from build123d import *

# Parameters (mm, degrees)
F0_W     = 1.5875
F0_H     = 19.05
F1_DEPTH = 30.48
F2_DEPTH = 19.6596
F4_DEPTH = 10.8204


with BuildPart() as f1:
    # F0 (on Front) → F1 (new body)
    with BuildSketch(Plane.XZ):
        with Locations((-5.55625, 10.795)):
            Rectangle(F0_W, F0_H)
        Polygon((-4.7625, 1.27), (-6.35, 1.27), (-6.35, -1.27), (6.35, -1.27), (6.35, 1.27), (4.7625, 1.27), align=None)
        with Locations((5.55625, 10.795)):
            Rectangle(F0_W, F0_H)
    extrude(amount=F1_DEPTH)

    # F1_face (on face) → F2 (cut)
    with BuildSketch(Plane(origin=(0, -30.48, 7.040217), x_dir=(1, 0, 0), z_dir=(0, -1, 0))):
        Polygon((-6.35, 13.279783), (-6.35, -8.310217), (6.35, -8.310217), (6.35, 13.279783), (4.7625, 13.279783), (4.7625, -5.770217), (-4.7625, -5.770217), (-4.7625, 13.279783), align=None)
    extrude(amount=-F2_DEPTH, mode=Mode.SUBTRACT)

    # F3 (on Front) → F4 (join)
    with BuildSketch(Plane.XZ):
        Polygon((-1.5875, 20.338782), (-3.175, 20.338782), (-3.175, 1.288782), (-3.175, 0), (-1.5875, 0), (-1.5875, 1.288782), align=None)
        Polygon((3.175, 20.338782), (1.5875, 20.338782), (1.5875, 1.288782), (1.5875, 0), (3.175, 0), (3.175, 1.288782), align=None)
    extrude(amount=F4_DEPTH)


solid = f1.part
Part model, mm, in its own coordinate system. A direction names the side the tool comes from. Give positions to 0.01 mm unless a question says otherwise; leave off trailing zeros. Loops run counter-clockwise (first coordinate to the right, second up) from the corner with the lowest first, then second, coordinate; pieces in that order, holes last. Notation, with made-up numbers: M 38.25,28 L 86.25,28 A38 cw 86.25,67 Z; hole C 88,-31 d3. An arc over 180 degrees is marked long. Put each result on its own line as item: value. Start each with the question number.
1) 3-axis set-ups, long thin cutter, end or side, ignore diameter. For faces 4 (the flat face through (-6, -5, 20.32)), 5 (the flat face through (4, -5, 1.27)), 6 (the flat face through (-2, -5, 20.339)), 7 (the flat face through (6, -5, 20.32)), 8 (the flat face through (-6.35, -5, 10)): which of +Z, -Z, +X, -X, +Y, -Y reach the whole face in a straight line?
2) Pull direction X, two halves, no side cores. Call faces 1 (the flat face through (-4, -5, 1.27)), 2 (the flat face through (6.35, -5, 9)), 3 (the flat face through (2, -5, 20.339)): +X half, -X half, draft (parallel to the pull), parting line (faces both ways), or undercut.
3) Probe probe 1 along Z at (x, y) = (6, -8.75); probe 2 along Z at (x, y) = (1.5, -7.5). List the from-to ranges inside material, lowest first.
4) Saw through at A-A (z = 18.5). State how many separate pieces and enclosed holes the cut face has, then the cut area to 3 significant figures.
5) Flat gauge pins, fed straight in: pin 1 (0.8 mm diameter, centred on x = 4, y = -7, fed in from +Z); pin 2 (1 mm diameter, centred on x = -5, y = -5, fed in from +Z). Where does each tip first touch, or does it go through?
6) Saw through at C-C (x = 4). List the corners of the cut face in (y, z).
Numbers:
1. face 4: +Z, -X, +Y, -Y
1. face 5: +Z, +Y, -Y
1. face 6: +Z, +X, -X, +Y, -Y
1. face 7: +Z, +X, +Y, -Y
1. face 8: +Z, -Z, -X, +Y, -Y
2. face 1: undercut
2. face 2: +X half
2. face 3: draft
3. probe 1: -1.27 to 20.32
3. probe 2: -1.27 to 1.27
4. separate pieces: 4
4. enclosed holes: 0
4. area: 68.7 mm^2
5. pin 1: z = 1.27
5. pin 2: z = 20.32
6. outline: M -10.82,-1.27 L 0,-1.27 L 0,1.27 L -10.82,1.27 Z
